Source: CAD feature listing. Evaluate the final solid. Frame: model axes, mm. A direction names the side the tool comes from. Give positions to 0.01 mm unless a question says otherwise; leave off trailing zeros. Order: outer loops, then holes, each group sorted by start corner. A loop starts at its lowest first (then second) coordinate and runs counter-clockwise, first axis right, second up. Notation, with made-up numbers: (-22.75, 48) - (16.25, 48) arc R30 ccw to (16.25, 72) - close; hole circle Ø4 at (9.5, 67). An arc over 180 degrees is marked (long way). Use CSV: the item, a comma, the result in double quotes.
```python
from build123d import *

# Parameters (mm, degrees)
BOSS_EXTRUDE1_DEPTH = 95
CUT_EXTRUDE1_DEPTH  = 124.177025455
BOSS_EXTRUDE2_DEPTH = 15
SKETCH4_W           = 50
SKETCH4_H           = 47.72
BOSS_EXTRUDE3_DEPTH = 20
SKETCH5_W           = 27
SKETCH5_H           = 47.72
BOSS_EXTRUDE4_DEPTH = 35


with BuildPart() as part:
    # Sketch1 → Boss-Extrude1 (new body)
    with BuildSketch(Plane(origin=(0, 0, 0), x_dir=(1, 0, 0), z_dir=(0, 1, 0))):
        with BuildLine():
            Line((-50.8, 22.86), (24.2, 22.86))
            Line((24.2, 22.86), (24.2, 15.5))
            Line((24.2, 15.5), (0, 15.5))
            ThreePointArc((0, 15.5), (-15.5, 0), (0, -15.5))
            Line((0, -15.5), (24.2, -15.5))
            Line((24.2, -15.5), (24.2, -22.86))
            Line((24.2, -22.86), (-50.8, -22.86))
            Line((-50.8, -22.86), (-50.8, 22.86))
        make_face()
    extrude(amount=BOSS_EXTRUDE1_DEPTH)

    # Sketch2 → Cut-Extrude1 (cut, through all)
    with BuildSketch(Plane(origin=(24.2, 0, 0), x_dir=(0, 0, -1), z_dir=(1, 0, 0))):
        Polygon((22.86, 0), (18.6436, 0), (22.86, 25.5524), align=None)
    extrude(amount=-CUT_EXTRUDE1_DEPTH, mode=Mode.SUBTRACT)

    # Sketch3 → Boss-Extrude2 (add)
    with BuildSketch(Plane(origin=(0, 95, 0), x_dir=(1, 0, 0), z_dir=(0, 1, 0))):
        with BuildLine():
            Line((24.2, 15.5), (24.2, 22.86))
            Line((24.2, 22.86), (-24.8, 22.86))
            Line((-24.8, 22.86), (-24.8, -22.86))
            Line((-24.8, -22.86), (24.2, -22.86))
            Line((24.2, -22.86), (24.2, -15.5))
            Line((24.2, -15.5), (0, -15.5))
            ThreePointArc((0, -15.5), (-15.5, 0), (0, 15.5))
            Line((0, 15.5), (24.2, 15.5))
        make_face()
    extrude(amount=BOSS_EXTRUDE2_DEPTH)

    # Sketch4 → Boss-Extrude3 (add)
    with BuildSketch(Plane(origin=(0, 110, 0), x_dir=(1, 0, 0), z_dir=(0, 1, 0))):
        with Locations((0.2, 0)):
            Rectangle(SKETCH4_W, SKETCH4_H)
    extrude(amount=BOSS_EXTRUDE3_DEPTH)

    # Sketch5 → Boss-Extrude4 (add)
    with BuildSketch(Plane(origin=(0, 95, 0), x_dir=(1, 0, 0), z_dir=(0, 1, 0))):
        with Locations((-38.3, 0)):
            Rectangle(SKETCH5_W, SKETCH5_H)
    extrude(amount=BOSS_EXTRUDE4_DEPTH)


solid = part.part
```
Item 1: First-contact query: pin 1 (1.1 mm diameter, centred on y = 100.5, z = -23.5, fed in from +X); pin 2 (4 mm diameter, centred on y = 36.5, z = 0, fed in from +X); pin 3 (22.5 mm diameter, centred on x = -22.5, y = 73, fed in from +Z). Flat tips, straight axial feed; report the tip coordinate or a pass-through.
Filled in:
pin 1,"stops at x = -24.8"
pin 2,"stops at x = -15.37"
pin 3,"stops at z = 22.86"
Item 2: Section A-A on z = 17.5. Return the cut outline in (x, y).
Filled in:
outline,"(-51.8, 95) - (-50.8, 95) - (-50.8, 0) - (24.2, 0) - (24.2, 110) - (25.2, 110) - (25.2, 130) - (-51.8, 130) - close"
Item 3: Material intervals for line 1 (Z direction, x = 10.5, y = 74); line 2 (Y direction, x = 19, z = -10); line 3 (X direction, y = 78, z = 17), sorted ascending. Write a range as from..to.
Filled in:
line 1,"z = -22.86..-15.5, 15.5..22.86"
line 2,"y = 110..130"
line 3,"x = -50.8..24.2"
Item 4: Section C-C on y = 64.5. Return the cut outline in (x, z).
Filled in:
outline,"(-50.8, -22.86) - (24.2, -22.86) - (24.2, -15.5) - (0, -15.5) arc R15.5 cw to (0, 15.5) - (24.2, 15.5) - (24.2, 22.86) - (-50.8, 22.86) - close"
Item 5: Set-up query: faces 5 (the flat face through (24.2, 54, 19)), 6 (the flat face through (12, 54, 15.5)), 7 (the flat face through (25.2, 120, 0)), 8 (the flat face through (-50.8, 47, 0)), 9 (the flat face through (-14, 130, 0)). Return all of +Z, -Z, +X, -X, +Y, -Y with unobstructed straight access to the full face (end or side cutting, diameter ignored); none if empty.
Filled in:
face 5,"+Z, -Z, +X, -Y"
face 6,"+X, -Y"
face 7,"+Z, -Z, +X, +Y, -Y"
face 8,"+Z, -Z, -X, -Y"
face 9,"+Z, -Z, +X, -X, +Y"
Item 6: Section D-D on x = -2. Return the cut outline in (y, z), then the cut area to 3 significant figures.
Filled in:
outline,"(0, -18.64) - (25.55, -22.86) - (110, -22.86) - (110, -23.86) - (130, -23.86) - (130, 23.86) - (110, 23.86) - (110, 22.86) - (0, 22.86) - (0, 15.37) - (110, 15.37) - (110, -15.37) - (0, -15.37) - close"
area,"2,550 mm2"
Item 7: Section B-B on x = -36.5. Return the cut outline in (y, z).
Filled in:
outline,"(0, -18.64) - (25.55, -22.86) - (95, -22.86) - (95, -23.86) - (130, -23.86) - (130, 23.86) - (95, 23.86) - (95, 22.86) - (0, 22.86) - close"
Item 8: Mould query, pull axis Z, two halves, no side actions, for faces 1 (the flat face through (-51, 95, 0)), 2 (the flat face through (12, 54, -15.5)), 3 (the flat face through (-12.775, 12.597, -20.722)), 4 (the flat face through (-22, 116, 23.86)). Classes: released by +Z, released by -Z, zero draft, split by the parting line, or undercut.
Filled in:
face 1,"zero draft"
face 2,"undercut"
face 3,"released by -Z"
face 4,"released by +Z"
